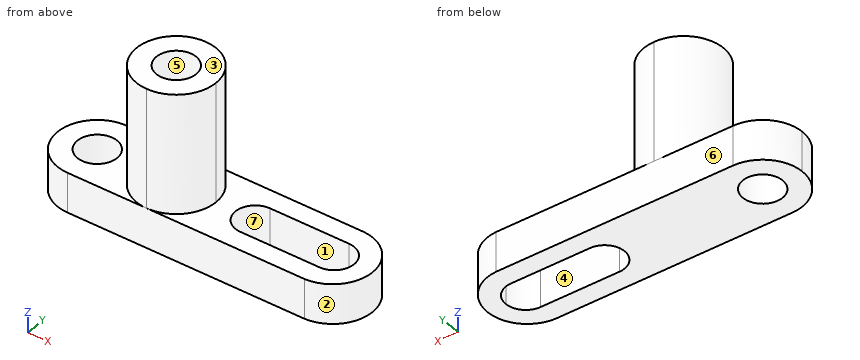
```python
from build123d import *

# Parameters (mm, degrees)
F0_W      = 101.6
F0_H      = 12.7
F1_DEPTH  = 25.4
F2_R      = 6.35
F3_DEPTH  = 25.4
F5_DEPTH  = 25.4
F7_DEPTH  = 25.4
F9_DEPTH  = 38.1
F10_R     = 6.35
F11_DEPTH = 38.1
F13_DEPTH = 25.4


# Not quite as in the source:
# - ends of sketch curves that miss each other by under 0.0002 mm in the source are joined


with BuildPart() as f1:
    # F0 (on Front) → F1 (new body)
    with BuildSketch(Plane.XZ):
        with Locations((50.8, 6.35)):
            Rectangle(F0_W, F0_H)
    extrude(amount=F1_DEPTH)

    # F2 (on face) → F3 (cut)
    with BuildSketch(Plane.XY.offset(12.7)):
        with Locations((12.7, -12.7)):
            Circle(F2_R)
    extrude(amount=-F3_DEPTH, mode=Mode.SUBTRACT)

    # F4 (on face) → F5 (cut)
    with BuildSketch(Plane.XY.offset(12.7)):
        with BuildLine():
            ThreePointArc((-1.0081e-06, -12.7), (3.7197432273, -3.7197435225), (12.7, 0))
            Line((12.7, 0), (0, 0))
            Line((0, 0), (-1.0081e-06, -12.7))
        make_face()
        with BuildLine():
            ThreePointArc((12.6999979839, -25.4), (3.7197425145, -21.6802557647), (-1.0081e-06, -12.7))
            Line((-1.0081e-06, -12.7), (0, -25.4))
            Line((0, -25.4), (12.6999979839, -25.4))
        make_face()
    extrude(amount=-F5_DEPTH, mode=Mode.SUBTRACT)

    # F6 (on face) → F7 (cut)
    with BuildSketch(Plane.XY.offset(12.7)):
        with BuildLine():
            ThreePointArc((63.5, -6.35), (67.9901280605, -8.2098719395), (69.85, -12.7))
            ThreePointArc((69.85, -12.7), (67.9901280605, -17.1901280605), (63.5, -19.05))
            Line((63.5, -19.05), (88.9, -19.05))
            ThreePointArc((88.9, -19.05), (82.55, -12.7), (88.9, -6.35))
            Line((88.9, -6.35), (63.5, -6.35))
        make_face()
        with BuildLine():
            ThreePointArc((63.5, -19.05), (67.9901280605, -17.1901280605), (69.85, -12.7))
            ThreePointArc((69.85, -12.7), (67.9901280605, -8.2098719395), (63.5, -6.35))
            ThreePointArc((63.5, -6.35), (57.15, -12.7), (63.5, -19.05))
        make_face()
        with BuildLine():
            ThreePointArc((95.25, -12.7), (93.3901280605, -8.2098719395), (88.9, -6.35))
            ThreePointArc((88.9, -6.35), (82.55, -12.7), (88.9, -19.05))
            ThreePointArc((88.9, -19.05), (93.3901280605, -17.1901280605), (95.25, -12.7))
        make_face()
    extrude(amount=-F7_DEPTH, mode=Mode.SUBTRACT)

    # F8 (on face) → F9 (join)
    with BuildSketch(Plane.XY.offset(12.7)):
        with BuildLine():
            ThreePointArc((38.1, -25.4), (47.0802561211, -21.6802561211), (50.8, -12.7))
            ThreePointArc((50.8, -12.7), (47.0802561211, -3.7197438789), (38.1, 0))
            ThreePointArc((38.1, 0), (25.4, -12.7), (38.1, -25.4))
        make_face()
    extrude(amount=F9_DEPTH)

    # F10 (on face) → F11 (cut)
    with BuildSketch(Plane.XY.offset(50.8)):
        with Locations((38.1, -12.7)):
            Circle(F10_R)
    extrude(amount=-F11_DEPTH, mode=Mode.SUBTRACT)

    # F12 (on face) → F13 (cut)
    with BuildSketch(Plane.XY.offset(12.7)):
        with BuildLine():
            ThreePointArc((88.9, 0), (101.1192301161, -12.7), (88.9, -25.4))
            Line((88.9, -25.4), (101.6, -25.4))
            Line((101.6, -25.4), (101.6, 0))
            Line((101.6, 0), (88.9, 0))
        make_face()
    extrude(amount=-F13_DEPTH, mode=Mode.SUBTRACT)


solid = f1.part
```
For this review, take the finished solid that the model builds, in its own axes (mm). Face numbers are marked on the shaded views. A direction names the side the tool comes from. Round coordinates to 2 decimals unless told otherwise and drop trailing zeros. Write each loop counter-clockwise with the first axis right and the second up, starting at its lowest first coordinate (ties: lowest second). Pieces come first, ordered by that corner, then holes. Notation, with made-up numbers: (9, -14.75) -> (43, -14.75) arc R18 ccw to (43, 2.25) -> close; hole circle Ø4 at (20, 65.5). An arc over 180 degrees is marked (long way). Use one line per item in the form item = value.
Q1. Clearance check with flat-ended pins moving along their axes: pin 1 Ø5 at (y, z) = (-13, 38) entering from -X; pin 2 Ø4 at (x, z) = (40.5, 24.5) entering from -Y; pin 3 Ø12 at (y, z) = (-15.5, 14) entering from -X; pin 4 Ø12 at (y, z) = (-21.5, 15) entering from +X. State where each tip first meets the part, or that it passes through.
Resolved:
pin_1 = 25.4
pin_2 = -25.39
pin_3 = 0
pin_4 = 100.69
Q2. To check wall thickness, follow probe 1 along Y at (x, z) = (64, 12); probe 2 along Z at (x, y) = (59, -0.75). State the ranges of each line that lie inside material, in increasing order. Write a range as from..to.
Resolved:
probe_1 = -25.4..-19.05, -6.35..0
probe_2 = 0..12.7
Q3. Consider section C-C (y = -9). State the section outline as (x, z) points, then the cut area to 3 significant figures.
Resolved:
outline = (0.55, 0) -> (7.54, 0) -> (7.54, 12.7) -> (0.55, 12.7) -> close; (17.86, 0) -> (58.34, 0) -> (58.34, 12.7) -> (50.25, 12.7) -> (50.25, 50.8) -> (43.26, 50.8) -> (43.26, 12.7) -> (32.94, 12.7) -> (32.94, 50.8) -> (25.95, 50.8) -> (25.95, 12.7) -> (17.86, 12.7) -> close; (94.06, 0) -> (100.57, 0) -> (100.57, 12.7) -> (94.06, 12.7) -> close
area = 1,220 mm²
Q4. Consider section D-D (x = 10.5). State the section outline as (y, z) points.
Resolved:
outline = (-25.21, 0) -> (-18.66, 0) -> (-18.66, 12.7) -> (-25.21, 12.7) -> close; (-6.74, 0) -> (-0.19, 0) -> (-0.19, 12.7) -> (-6.74, 12.7) -> close
Q5. Machinability: for the marked faces 5, 6 and 7, which of the approach directions +Z, -Z, +X, -X, +Y, -Y give a long, thin tool a straight path to every point of the face, cutting with its end or side? Answer none if there is none.
Resolved:
face_5 = +Z
face_6 = +Z, -Z, +X, -X, +Y
face_7 = +Z, -Z
Q6. Consider section A-A (x = 77.5). State the section outline as (y, z) points, then the cut area to 3 significant figures.
Resolved:
outline = (-25.4, 0) -> (-19.05, 0) -> (-19.05, 12.7) -> (-25.4, 12.7) -> close; (-6.35, 0) -> (0, 0) -> (0, 12.7) -> (-6.35, 12.7) -> close
area = 161 mm²
Q7. Consider section B-B (z = 11). State the section outline as (x, y) points, then the cut area to 3 significant figures.
Resolved:
outline = (12.7, -25.4) -> (88.9, -25.4) arc R12.71 ccw to (88.9, 0) -> (12.7, 0) arc R12.7 ccw to start; hole circle Ø12.7 at (12.7, -12.7); hole (63.5, -19.05) -> (88.9, -19.05) arc R6.35 ccw to (88.9, -6.35) -> (63.5, -6.35) arc R6.35 ccw to start
area = 1,850 mm²
Q8. The part is to be moulded in two halves that separate along X. For the marked faces 1, 2, 3 and 4, say which applies: released by +X, released by -X, zero draft, split by the parting line, or undercut.
Resolved:
face_1 = undercut
face_2 = released by +X
face_3 = zero draft
face_4 = undercut
